from build123d import *

# Parameters (mm, degrees)
SKETCH1_R           = 2.8702
BOSS_EXTRUDE1_DEPTH = 6.35
FILLET1_R           = 9
FILLET2_R           = 9


with BuildPart() as part:
    # Sketch1 → Boss-Extrude1 (new body)
    with BuildSketch(Plane.XY):
        Polygon((-38.642090152, 26.982634823), (-45.206950064, 26.982634823), (-45.206950064, 71.432634823), (-61.6, 71.432634823), (-61.6, 14.282634823), (-45.206950064, 14.282634823), (-38.642090152, 14.282634823), align=None)
        with Locations((-53.575, 59.289941788)):
            Circle(SKETCH1_R, mode=Mode.SUBTRACT)
    extrude(amount=BOSS_EXTRUDE1_DEPTH)

    # Fillet1
    # the kernel refuses this fillet: 9 mm, written as the material it takes off along each edge
    with BuildSketch(Plane(origin=(-45.206950064, 71.432634823, -22.5), x_dir=(-1, 0, 0), z_dir=(0, 0, 1)), Plane(origin=(-61.6, 71.432634823, -22.5), x_dir=(0, -1, 0), z_dir=(0, 0, 1))) as fillet1_piece_1:
        with BuildLine():
            CenterArc((FILLET1_R, FILLET1_R), FILLET1_R, 180, 90)
            Line((0, FILLET1_R), (0, 0))
            Line((0, 0), (FILLET1_R, 0))
        make_face()
    extrude(amount=51.35, mode=Mode.SUBTRACT)

    # Fillet2
    fillet2_edges = [part.edges().sort_by_distance(p)[0] for p in [
        (-61.6, 14.282634823, 3.175),
    ]]
    fillet(fillet2_edges, radius=FILLET2_R)


solid = part.part
Build history of the part. All positions in model axes, mm. A direction names the side the tool comes from. Give positions to 0.01 mm unless a question says otherwise; leave off trailing zeros. Order: outer loops, then holes, each group sorted by start corner. A loop starts at its lowest first (then second) coordinate and runs counter-clockwise, first axis right, second up. Notation, with made-up numbers: M 49,12.25 L 80,12.25 A13 cw 80,26.25 Z; hole C 7,-24 d10. An arc over 180 degrees is marked long. Use one line per item in the form item = value.
1) Tool access for faces 4 (the face through (-42, 26.983, 3)), 5 (the face through (-59.179, 68.574, 3.131)): list every direction of +Z, -Z, +X, -X, +Y, -Y with a clear straight run to the whole face (end or side of a thin tool).
Calculated:
face_4 = +Z, -Z, +X, +Y
face_5 = +Z, -Z, -X, +Y
2) Two-plate mould, pull along Y, no slides. Class faces 1 (the face through (-45.207, 44, 3)), 2 (the face through (-47.502, 68.437, 3.131)), 3 (the face through (-54.2, 56.49, 3.13)): released by +Y, released by -Y, zero draft, split by the parting line, or undercut.
Calculated:
face_1 = zero draft
face_2 = released by +Y
face_3 = undercut
3) Saw through at B-B (x = -41.75). Give the cut face in (y, z), plus the area to 3 significant figures.
Calculated:
outline = M 14.28,0 L 26.98,0 L 26.98,6.35 L 14.28,6.35 Z
area = 80.6 mm2
4) Drop a flat-ended pin along its axis: pin 1 (1 mm diameter, centred on y = 46.5, z = 0.5, fed in from +X). Give the stop position or say it passes through.
Calculated:
pin_1 = -45.21
5) Saw through at A-A (z = 4.25). Give the cut face in (x, y) (3 decimals), plus the area to 3 significant figures.
Calculated:
outline = M -61.6,23.283 A9 ccw -52.6,14.283 L -38.642,14.283 L -38.642,26.983 L -45.207,26.983 L -45.207,62.433 A9 ccw -53.403,71.397 A9 ccw -61.6,62.433 Z; hole C -53.575,59.29 d5.74
area = 942 mm2
6) Saw through at C-C (y = 50.5). Give the cut face in (x, z), plus the area to 3 significant figures.
Calculated:
outline = M -61.6,0 L -45.21,0 L -45.21,6.35 L -61.6,6.35 Z
area = 104 mm2
7) Probe probe 1 along X at (y, z) = (59.5, 6.25); probe 2 along Y at (x, z) = (-42.25, 2.75); probe 3 along X at (y, z) = (38.5, 2.5). List the from-to ranges inside material, lowest first.
Calculated:
probe_1 = -61.6 to -56.44, -50.71 to -45.21
probe_2 = 14.28 to 26.98
probe_3 = -61.6 to -45.21
